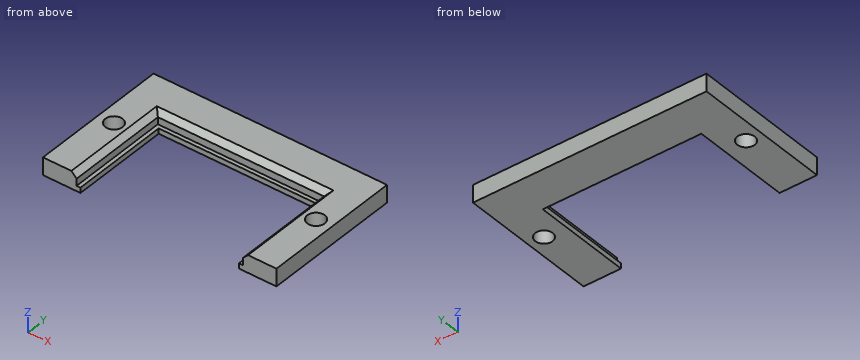
from build123d import *

# Parameters (mm, degrees)
SKETCH_W        = 67
SKETCH_H        = 40
PAD_DEPTH       = 5
SKETCH001_W     = 45.5
SKETCH001_H     = 28.3
POCKET_DEPTH    = 5.001
SKETCH002_W     = 47.7
SKETCH002_H     = 29.4
POCKET001_DEPTH = 3.5
SKETCH003_R     = 2.5
POCKET002_DEPTH = 5.001
CHAMFER_SIZE    = 1.5


with BuildPart() as part:
    # Sketch → Pad (new body)
    with BuildSketch(Plane.XY):
        Rectangle(SKETCH_W, SKETCH_H)
    extrude(amount=PAD_DEPTH)

    # Sketch001 (on Face6 of Pad) → Pocket (cut, through all)
    with BuildSketch(Plane.XY.offset(5)):
        with Locations((0, -5.85)):
            Rectangle(SKETCH001_W, SKETCH001_H)
    extrude(amount=-POCKET_DEPTH, mode=Mode.SUBTRACT)

    # Sketch002 (on Face5 of Pocket) → Pocket001 (cut)
    with BuildSketch(Plane.XY.offset(5)):
        with Locations((0, -5.3)):
            Rectangle(SKETCH002_W, SKETCH002_H)
    extrude(amount=-POCKET001_DEPTH, mode=Mode.SUBTRACT)

    # Sketch003 (on Face5 of Pocket001) → Pocket002 (cut, through all)
    with BuildSketch(Plane.XY.offset(5)):
        with Locations((29, 0)):
            Circle(SKETCH003_R)
        with Locations((-29, 0)):
            Circle(SKETCH003_R)
    extrude(amount=-POCKET002_DEPTH, mode=Mode.SUBTRACT)

    # Chamfer
    chamfer_edges = [part.edges().sort_by_distance(p)[0] for p in [
        (0, 9.4, 5),
        (-23.85, -5.3, 5),
        (23.85, -5.3, 5),
    ]]
    chamfer(chamfer_edges, length=CHAMFER_SIZE)


solid = part.part
The model under review builds one solid part; all positions refer to its coordinate system, in mm. Round coordinates to 2 decimals unless told otherwise and drop trailing zeros. Loops run counter-clockwise (first coordinate to the right, second up) from the corner with the lowest first, then second, coordinate; pieces in that order, holes last. Notation, with made-up numbers: (6, 37.5) -> (42, 37.5) arc R23 ccw to (42, 51.5) -> close; hole circle Ø11 at (12.5, 81.25). An arc over 180 degrees is marked (long way). One line per question, with ' | ' between items. Start each with the question number.
Item 1: Add section C-C, the plane x = -29. Write out the cut boundary in (y, z), then the cut area to 3 significant figures.
Item 2: Add section D-D, the plane z = 2.35. Write out the cut boundary in (x, y), then the cut area to 3 significant figures.
Item 3: Wall thickness on line 1 along X through (y, z) = (-9.5, 1.95); line 2 along X through (y, z) = (-7, 1.15); line 3 along Y through (x, z) = (29, 3.9): over which ranges is each line inside the solid? List them lowest first. Write a range as [from, to].
Item 4: Add section A-A, the plane y = -9. Write out the cut boundary in (x, z).
Item 5: For pin 1 (1.6 mm diameter, centred on x = -6, z = 3, fed in from -Y), flat-tipped, find the tip position at first contact; note if it passes through.
Item 6: Add section B-B, the plane y = 0. Write out the cut boundary in (x, z), then the cut area to 4 significant figures.
Return value:
1) outline: (-20, 0) -> (-2.5, 0) -> (-2.5, 5) -> (-20, 5) -> close; (2.5, 0) -> (20, 0) -> (20, 5) -> (2.5, 5) -> close | area: 175 mm2
2) outline: (-33.5, -20) -> (-23.85, -20) -> (-23.85, 9.4) -> (23.85, 9.4) -> (23.85, -20) -> (33.5, -20) -> (33.5, 20) -> (-33.5, 20) -> close; hole circle Ø5 at (-29, 0); hole circle Ø5 at (29, 0) | area: 1,240 mm2
3) line 1: x = [-33.5, -23.85], [23.85, 33.5] | line 2: x = [-33.5, -22.75], [22.75, 33.5] | line 3: y = [-20, -2.5], [2.5, 20]
4) outline: (-33.5, 0) -> (-22.75, 0) -> (-22.75, 1.5) -> (-23.85, 1.5) -> (-23.85, 3.5) -> (-25.35, 5) -> (-33.5, 5) -> close; (22.75, 0) -> (33.5, 0) -> (33.5, 5) -> (25.35, 5) -> (23.85, 3.5) -> (23.85, 1.5) -> (22.75, 1.5) -> close
5) pin 1: stops at y = 9.4
6) outline: (-33.5, 0) -> (-31.5, 0) -> (-31.5, 5) -> (-33.5, 5) -> close; (-26.5, 0) -> (-22.75, 0) -> (-22.75, 1.5) -> (-23.85, 1.5) -> (-23.85, 3.5) -> (-25.35, 5) -> (-26.5, 5) -> close; (22.75, 0) -> (26.5, 0) -> (26.5, 5) -> (25.35, 5) -> (23.85, 3.5) -> (23.85, 1.5) -> (22.75, 1.5) -> close; (31.5, 0) -> (33.5, 0) -> (33.5, 5) -> (31.5, 5) -> close | area: 47.55 mm2
